Check sheet for the modelled part. Datum: model origin and axes. Units: mm. Face numbers are marked on the shaded views. A direction names the side the tool comes from. Coordinates: 2 decimals unless noted, no trailing zeros. Loops run counter-clockwise (first coordinate to the right, second up) from the corner with the lowest first, then second, coordinate; pieces in that order, holes last. Notation, with made-up numbers: (-21, 49.25) - (17, 49.25) arc R16 ccw to (17, 70.25) - close; hole circle Ø4 at (-24, -5.75). An arc over 180 degrees is marked (long way). Write each question's results on one line, items separated by ' | '. Start each with the question number.
1. Cross-section at B-B (x = -9). Record the cut outline in (y, z), and give its area (3 significant figures).
2. Tool access check on the marked faces 4, 5 and 6. Record the directions out of +Z, -Z, +X, -X, +Y, -Y that give a thin tool (end or side, any length) a straight path to the whole face; none if there is none.
3. Draft check along X on the marked faces 1, 2 and 3. Enter one of: released by +X, released by -X, zero draft, split by the parting line, or undercut.
4. Cross-section at A-A (y = -7.95). Record the cut outline in (x, z), and give its area (3 significant figures).
5. Thickness scan on line 1 (X direction, y = 0, z = 16.5); line 2 (X direction, y = 15, z = 4.75); line 3 (Y direction, x = 9, z = 1.8). Record the ranges inside material, lowest first. Write a range as [from, to].
6. Gauge pin test, flat ends, axial feed: P1, Ø8, axis at x = 0, y = -18, coming from the +Z side; P2, Ø3, axis at x = 43, z = 7, coming from the -Y side; P3, Ø3, axis at x = -6, z = 11, coming from the +Y side; P4, Ø3, axis at x = -13.77, y = -7.95, coming from the +Z side. Record the tip position at first contact, or that the pin passes through.
7. Cross-section at C-C (z = 18). Give the number of separate pieces and of enclosed holes in the cut face, and give its area (3 significant figures).
```python
from build123d import *

# Parameters (mm, degrees)
SKETCH1_R           = 45
BOSS_EXTRUDE1_DEPTH = 5
SKETCH2_R           = 2.5
CUT_EXTRUDE1_DEPTH  = 5
SKETCH3_R           = 45
SKETCH3_R_2         = 43
BOSS_EXTRUDE2_DEPTH = 10
SKETCH4_R           = 60
SKETCH4_R_2         = 43
BOSS_EXTRUDE3_DEPTH = 5
SKETCH5_R           = 2
CUT_EXTRUDE2_DEPTH  = 5
CUT_EXTRUDE3_START  = 30
CUT_EXTRUDE3_DEPTH  = 81
SKETCH7_R           = 35
SKETCH7_R_2         = 2.5
BOSS_EXTRUDE4_DEPTH = 7.5


with BuildPart() as part:
    # Sketch1 → Boss-Extrude1 (new body)
    with BuildSketch(Plane.XY):
        Circle(SKETCH1_R)
    extrude(amount=BOSS_EXTRUDE1_DEPTH)

    # Sketch2 → Cut-Extrude1 (cut)
    with BuildSketch(Plane.XY.offset(5)):
        with Locations((0, 15.9)):
            Circle(SKETCH2_R)
        with Locations((13.76980392, -7.95)):
            Circle(SKETCH2_R)
        with Locations((-13.76980392, -7.95)):
            Circle(SKETCH2_R)
        with Locations((9, 15.588457268)):
            Circle(SKETCH2_R)
        with Locations((15.588457268, 9)):
            Circle(SKETCH2_R)
        with Locations((18, 0)):
            Circle(SKETCH2_R)
        with Locations((9, -15.588457268)):
            Circle(SKETCH2_R)
        with Locations((0, -18)):
            Circle(SKETCH2_R)
        with Locations((-9, -15.588457268)):
            Circle(SKETCH2_R)
        with Locations((-18, 0)):
            Circle(SKETCH2_R)
        with Locations((-15.588457268, 9)):
            Circle(SKETCH2_R)
        with Locations((-9, 15.588457268)):
            Circle(SKETCH2_R)
    extrude(amount=-CUT_EXTRUDE1_DEPTH, mode=Mode.SUBTRACT)

    # Sketch3 → Boss-Extrude2 (add)
    with BuildSketch(Plane.XY.offset(5)):
        Circle(SKETCH3_R)
        Circle(SKETCH3_R_2, mode=Mode.SUBTRACT)
    extrude(amount=BOSS_EXTRUDE2_DEPTH)

    # Sketch4 → Boss-Extrude3 (add)
    with BuildSketch(Plane.XY.offset(15)):
        Circle(SKETCH4_R)
        Circle(SKETCH4_R_2, mode=Mode.SUBTRACT)
    extrude(amount=BOSS_EXTRUDE3_DEPTH)

    # Sketch5 → Cut-Extrude2 (cut)
    with BuildSketch(Plane.XY.offset(20)):
        with Locations((0, 53)):
            Circle(SKETCH5_R)
        with Locations((31.274207169, 43.143144086)):
            Circle(SKETCH5_R)
        with Locations((50.527584161, 16.643144086)):
            Circle(SKETCH5_R)
        with Locations((50.527584161, -16.112657318)):
            Circle(SKETCH5_R)
        with Locations((31.274207169, -42.612657318)):
            Circle(SKETCH5_R)
        with Locations((0.121588798, -52.734756616)):
            Circle(SKETCH5_R)
        with Locations((-31.031029574, -42.612657318)):
            Circle(SKETCH5_R)
        with Locations((-50.284406566, -16.112657318)):
            Circle(SKETCH5_R)
        with Locations((-50.284406566, 16.643144086)):
            Circle(SKETCH5_R)
        with Locations((-31.031029574, 43.143144086)):
            Circle(SKETCH5_R)
    extrude(amount=-CUT_EXTRUDE2_DEPTH, mode=Mode.SUBTRACT)

    # Sketch6 → Cut-Extrude3 (cut)
    with BuildSketch(Plane(origin=(0, 0, 0), x_dir=(1, 0, 0), z_dir=(0, 1, 0)).offset(CUT_EXTRUDE3_START)):
        Polygon((-25, -15), (-25, 5), (25, 5), (25, -15), (25, -26.812611245), (-25, -26.812611245), align=None)
    extrude(amount=CUT_EXTRUDE3_DEPTH, mode=Mode.SUBTRACT)

    # Sketch7 → Boss-Extrude4 (add)
    with BuildSketch(Plane(origin=(0, 0, 0), x_dir=(-1, 0, 0), z_dir=(0, 0, -1))):
        with Locations(Location((0, 0, 0), (0, 0, 121.002719134))):
            Circle(SKETCH7_R)
        with Locations(Location((-15.588457268, 9, 0), (0, 0, 180))):
            Circle(SKETCH7_R_2, mode=Mode.SUBTRACT)
        with Locations(Location((-18, 0, 0), (0, 0, 180))):
            Circle(SKETCH7_R_2, mode=Mode.SUBTRACT)
        with Locations(Location((-13.76980392, -7.95, 0), (0, 0, 180))):
            Circle(SKETCH7_R_2, mode=Mode.SUBTRACT)
        with Locations(Location((-9, -15.588457268, 0), (0, 0, 180))):
            Circle(SKETCH7_R_2, mode=Mode.SUBTRACT)
        with Locations(Location((0, -18, 0), (0, 0, 180))):
            Circle(SKETCH7_R_2, mode=Mode.SUBTRACT)
        with Locations(Location((9, -15.588457268, 0), (0, 0, 180))):
            Circle(SKETCH7_R_2, mode=Mode.SUBTRACT)
        with Locations(Location((13.76980392, -7.95, 0), (0, 0, 180))):
            Circle(SKETCH7_R_2, mode=Mode.SUBTRACT)
        with Locations(Location((18, 0, 0), (0, 0, 180))):
            Circle(SKETCH7_R_2, mode=Mode.SUBTRACT)
        with Locations(Location((15.588457268, 9, 0), (0, 0, 180))):
            Circle(SKETCH7_R_2, mode=Mode.SUBTRACT)
        with Locations(Location((9, 15.588457268, 0), (0, 0, 180))):
            Circle(SKETCH7_R_2, mode=Mode.SUBTRACT)
        with Locations(Location((0, 15.9, 0), (0, 0, 180))):
            Circle(SKETCH7_R_2, mode=Mode.SUBTRACT)
        with Locations(Location((-9, 15.588457268, 0), (0, 0, 180))):
            Circle(SKETCH7_R_2, mode=Mode.SUBTRACT)
    extrude(amount=BOSS_EXTRUDE4_DEPTH)


solid = part.part
```
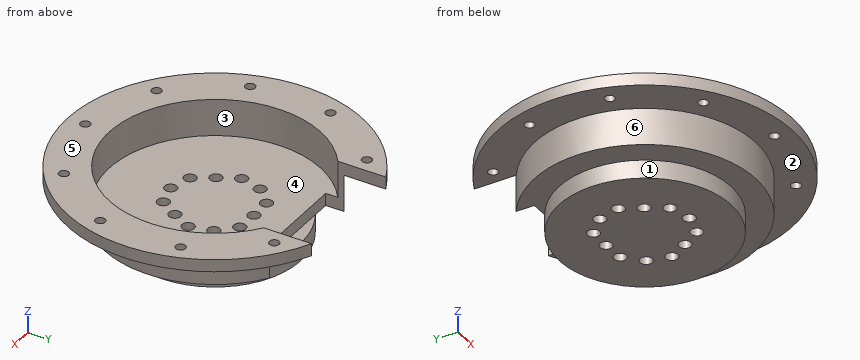
Established:
1) outline: (-59.32, 15) - (-44.09, 15) - (-44.09, 0) - (-33.82, 0) - (-33.82, -7.5) - (-18.09, -7.5) - (-18.09, 5) - (-42.05, 5) - (-42.05, 20) - (-59.32, 20) - close; (-13.09, -7.5) - (13.09, -7.5) - (13.09, 5) - (-13.09, 5) - close; (18.09, -7.5) - (33.82, -7.5) - (33.82, 0) - (30, 0) - (30, 5) - (18.09, 5) - close | area: 860 mm^2
2) face 4: +Z | face 5: +Z, +X, -X, +Y, -Y | face 6: -Z
3) face 1: split by the parting line | face 2: zero draft | face 3: undercut
4) outline: (-59.47, 15) - (-44.29, 15) - (-44.29, 0) - (-34.09, 0) - (-34.09, -7.5) - (-16.27, -7.5) - (-16.27, 5) - (-42.26, 5) - (-42.26, 20) - (-59.47, 20) - close; (-11.27, -7.5) - (11.27, -7.5) - (11.27, 5) - (-11.27, 5) - close; (16.27, -7.5) - (34.09, -7.5) - (34.09, 0) - (44.29, 0) - (44.29, 15) - (59.47, 15) - (59.47, 20) - (42.26, 20) - (42.26, 5) - (16.27, 5) - close | area: 1,040 mm^2
5) line 1: [-60, -43], [43, 60] | line 2: [-42.43, -11.43], [-6.57, -2.33], [2.33, 6.57], [11.43, 42.43] | line 3: [-44.09, -18.09], [-13.09, 13.09], [18.09, 30]
6) P1: z = 5 | P2: y = -17.4 | P3: y = -42.34 | P4: through
7) separate pieces: 1 | enclosed holes: 9 | area: 4,500 mm^2
